from build123d import *
from OCP.BRepFilletAPI import BRepFilletAPI_MakeChamfer

# Parameters (mm, degrees)
BOSS_EXTRUDE1_DEPTH            = 7.5
CUT_EXTRUDE1_REACH             = 58.013
SKETCH2_R                      = 1
CUT_EXTRUDE1_DIRECTION_2_DEPTH = 57.013391256
CHAMFER1_SIZE                  = 5
CHAMFER1_SIZE2                 = 4.351474633
CUT_EXTRUDE2_REACH             = 57.607
SKETCH3_R                      = 13.75
SKETCH11_W                     = 45
SKETCH11_H                     = 7.5
BOSS_EXTRUDE2_DEPTH            = 5
M4_TAPPED_HOLE1_D              = 3.3
CUT_EXTRUDE3_REACH             = 57.607
SKETCH6_R                      = 4.1
M4_TAPPED_HOLE2_REACH          = 61.725
M4_TAPPED_HOLE2_BORE_R         = 1.65
M3_TAPPED_HOLE1_AT_2_COUNT     = 2
M3_TAPPED_HOLE1_AT_2_PITCH     = 12


with BuildPart() as part:
    # Sketch1 → Boss-Extrude1 (new body)
    with BuildSketch(Plane(origin=(0, 0, 0), x_dir=(1, 0, 0), z_dir=(0, 1, 0))):
        Polygon((-22.5, 0), (22.5, 0), (22.5, 14.6), (27.5, 14.6), (32.5, 45), (-32.5, 45), (-27.5, 14.6), (-22.5, 14.6), align=None)
    extrude(amount=BOSS_EXTRUDE1_DEPTH)

    # Sketch2 → Cut-Extrude1 (cut, up to next)
    with BuildSketch(Plane(origin=(0, 7.5, 0), x_dir=(1, 0, 0), z_dir=(0, 1, 0)), mode=Mode.PRIVATE) as cut_extrude1_sk1:
        with Locations((-23.5, 14.6)):
            Circle(SKETCH2_R)
    cut_extrude1_tool1 = extrude(cut_extrude1_sk1.sketch, amount=-CUT_EXTRUDE1_REACH, mode=Mode.PRIVATE) & part.part
    # Sketch2 → Cut-Extrude1 (cut, up to next)
    with BuildSketch(Plane(origin=(0, 7.5, 0), x_dir=(1, 0, 0), z_dir=(0, 1, 0)), mode=Mode.PRIVATE) as cut_extrude1_sk2:
        with Locations((23.5, 14.6)):
            Circle(SKETCH2_R)
    cut_extrude1_tool2 = extrude(cut_extrude1_sk2.sketch, amount=-CUT_EXTRUDE1_REACH, mode=Mode.PRIVATE) & part.part
    add(cut_extrude1_tool1.solids().sort_by_distance((-23.5, 7.5, -14.6))[0], mode=Mode.SUBTRACT)
    add(cut_extrude1_tool2.solids().sort_by_distance((23.5, 7.5, -14.6))[0], mode=Mode.SUBTRACT)

    # Sketch2 → Cut-Extrude1 direction 2 (cut)
    with BuildSketch(Plane(origin=(0, 7.5, 0), x_dir=(1, 0, 0), z_dir=(0, 1, 0))):
        with Locations((-23.5, 14.6)):
            Circle(SKETCH2_R)
        with Locations((23.5, 14.6)):
            Circle(SKETCH2_R)
    extrude(amount=CUT_EXTRUDE1_DIRECTION_2_DEPTH, mode=Mode.SUBTRACT)

    # Chamfer1: one chamfer whose edges measure the first distance from different faces: ONE call of the kernel's chamfer builder (chamfer() names one face for all edges)
    chamfer1_edges_1 = [part.edges().sort_by_distance(p)[0] for p in [
        (-32.5, 3.75, -45),
    ]]
    chamfer1_side_1 = [part.faces().sort_by_distance(p)[0] for p in [
        (0, 3.75, -45),
    ]]
    chamfer1_edges_2 = [part.edges().sort_by_distance(p)[0] for p in [
        (32.5, 3.75, -45),
    ]]
    chamfer1_side_2 = [part.faces().sort_by_distance(p)[0] for p in [
        (30, 3.75, -29.8),
    ]]
    chamfer1 = BRepFilletAPI_MakeChamfer(part.part.solid().wrapped)
    for e in chamfer1_edges_1:
        chamfer1.Add(CHAMFER1_SIZE, CHAMFER1_SIZE2, e.wrapped, chamfer1_side_1[0].wrapped)  # the first distance lies on this face
    for e in chamfer1_edges_2:
        chamfer1.Add(CHAMFER1_SIZE, CHAMFER1_SIZE2, e.wrapped, chamfer1_side_2[0].wrapped)  # the first distance lies on this face
    add(Compound.cast(chamfer1.Shape()), mode=Mode.REPLACE)

    # Sketch3 → Cut-Extrude2 (cut, up to next)
    with BuildSketch(Plane(origin=(0, 7.5, 0), x_dir=(1, 0, 0), z_dir=(0, 1, 0)), mode=Mode.PRIVATE) as cut_extrude2_sk1:
        with Locations(Location((0, 21, 0), (0, 0, 270))):
            Circle(SKETCH3_R)
    cut_extrude2_tool1 = extrude(cut_extrude2_sk1.sketch, amount=-CUT_EXTRUDE2_REACH, mode=Mode.PRIVATE) & part.part
    add(cut_extrude2_tool1.solids().sort_by_distance((0, 7.5, -21))[0], mode=Mode.SUBTRACT)

    # Sketch11 → Boss-Extrude2 (add)
    with BuildSketch(Plane.XY):
        with Locations((0, 3.75)):
            Rectangle(SKETCH11_W, SKETCH11_H)
    extrude(amount=BOSS_EXTRUDE2_DEPTH)

    # M4 Tapped Hole1 (through all)
    with Locations(Plane(origin=(0, 0, 0), x_dir=(-1, 0, 0), z_dir=(0, -1, 0))):
        with Locations((-18.3, 21), (18.3, 21)):
            Hole(M4_TAPPED_HOLE1_D / 2)

    # Sketch6 → Cut-Extrude3 (cut, up to next)
    with BuildSketch(Plane.XZ, mode=Mode.PRIVATE) as cut_extrude3_sk1:
        with Locations(Location((18.5, -28.5, 0), (0, 0, 270))):
            Circle(SKETCH6_R)
    cut_extrude3_tool1 = extrude(cut_extrude3_sk1.sketch, amount=-CUT_EXTRUDE3_REACH, mode=Mode.PRIVATE) & part.part
    # Sketch6 → Cut-Extrude3 (cut, up to next)
    with BuildSketch(Plane.XZ, mode=Mode.PRIVATE) as cut_extrude3_sk2:
        with Locations(Location((-18.5, -28.5, 0), (0, 0, 270))):
            Circle(SKETCH6_R)
    cut_extrude3_tool2 = extrude(cut_extrude3_sk2.sketch, amount=-CUT_EXTRUDE3_REACH, mode=Mode.PRIVATE) & part.part
    add(cut_extrude3_tool1.solids().sort_by_distance((18.5, 0, -28.5))[0], mode=Mode.SUBTRACT)
    add(cut_extrude3_tool2.solids().sort_by_distance((-18.5, 0, -28.5))[0], mode=Mode.SUBTRACT)

    # M4 Tapped Hole2 bore → M4 Tapped Hole2 (cut, up to next)
    with BuildSketch(Plane(origin=(0, 0, -45), x_dir=(-1, 0, 0), z_dir=(0, 0, -1)), mode=Mode.PRIVATE) as m4_tapped_hole2_sk1:
        with Locations((-18.5, 3.75)):
            Circle(M4_TAPPED_HOLE2_BORE_R)
    m4_tapped_hole2_tool1 = extrude(m4_tapped_hole2_sk1.sketch, amount=-M4_TAPPED_HOLE2_REACH, mode=Mode.PRIVATE) & part.part
    # M4 Tapped Hole2 bore → M4 Tapped Hole2 (cut, up to next)
    with BuildSketch(Plane(origin=(0, 0, -45), x_dir=(-1, 0, 0), z_dir=(0, 0, -1)), mode=Mode.PRIVATE) as m4_tapped_hole2_sk2:
        with Locations((18.5, 3.75)):
            Circle(M4_TAPPED_HOLE2_BORE_R)
    m4_tapped_hole2_tool2 = extrude(m4_tapped_hole2_sk2.sketch, amount=-M4_TAPPED_HOLE2_REACH, mode=Mode.PRIVATE) & part.part
    add(m4_tapped_hole2_tool1.solids().sort_by_distance((18.5, 3.75, -45))[0], mode=Mode.SUBTRACT)
    add(m4_tapped_hole2_tool2.solids().sort_by_distance((-18.5, 3.75, -45))[0], mode=Mode.SUBTRACT)

    # Sketch10 → M3 Tapped Hole1 (revolve, cut)
    with BuildSketch(Plane(origin=(22.5, 3.75, -10.5), x_dir=(0, 0, -1), z_dir=(0, 1, 0))):
        Polygon((0, 0), (0, 10.751075774), (1.25, 10), (1.25, 0), align=None)
    m3_tapped_hole1 = revolve(axis=Axis((28.85, 3.75, -10.5), (-1, 0, 0)), mode=Mode.SUBTRACT)

    # M3 Tapped Hole1 at 2: M3 Tapped Hole1 ×2
    with Locations(*[(0, 0, i * M3_TAPPED_HOLE1_AT_2_PITCH) for i in range(1, M3_TAPPED_HOLE1_AT_2_COUNT)]):
        add(m3_tapped_hole1, mode=Mode.SUBTRACT)

    # Mirror1: M3 Tapped Hole1 across plane
    add(m3_tapped_hole1.mirror(Plane(origin=(0, 0, 0), x_dir=(0, 0, 1), z_dir=(1, 0, 0))), mode=Mode.SUBTRACT)

    # Mirror1 copy 1 sketch → Mirror1 copy 1 (revolve, cut)
    with BuildSketch(Plane(origin=(-22.5, 3.75, 1.5), x_dir=(0, 0, -1), z_dir=(0, 1, 0))):
        Polygon((0, 0), (0, -10.751075774), (1.25, -10), (1.25, 0), align=None)
    revolve(axis=Axis((-28.85, 3.75, 1.5), (-1, 0, 0)), mode=Mode.SUBTRACT)


solid = part.part
Can you work these out from the model? Positions are in its coordinate system, mm. A direction names the side the tool comes from. Round coordinates to 2 decimals unless told otherwise and drop trailing zeros. Write each loop counter-clockwise with the first axis right and the second up, starting at its lowest first coordinate (ties: lowest second). Pieces come first, ordered by that corner, then holes. Notation, with made-up numbers: (3, 46.25) - (47, 46.25) arc R17 ccw to (47, 57.25) - close; hole circle Ø9 at (-28, 65.5). An arc over 180 degrees is marked (long way). Write each question's results on one line, items separated by ' | '. Start each with the question number.
1) Please list where these lines run through material, in increasing order: line 1 (X direction, y = 1.5, z = -20); line 2 (X direction, y = 4.25, z = -21); line 3 (Z direction, x = -18.3, y = 2.75).
2) Suppose I cut it at D-D (z = -8.5). List the corners of the cut face in (x, y) for me.
3) We'd pull the mould along X, two halves only. Please class faces 4 (the flat face through (-29.677, 3.698, -27.836)), 5 (the cylindrical face through (23.5, 3.8, -15.6)), 6 (the flat face through (-15, 0, -20)): released by +X, released by -X, zero draft, split by the parting line, or undercut.
4) Suppose I cut it at A-A (x = 0). List the corners of the cut face in (y, z) for me.
5) Suppose I cut it at B-B (z = -30). List the corners of the cut face in (x, y) for me, and give its area (3 significant figures).
6) Which directions (+Z, -Z, +X, -X, +Y, -Y) give clear straight access to the entire face, cutting with the end or side of a thin tool? Please do faces 1 (the flat face through (-22.5, 4, -5)), 2 (the cylindrical face through (19.81, 2.75, -38.72)), 3 (the cylindrical face through (-17.57, 3.7, -9.25)).
7) Suppose I cut it at C-C (x = 18.5). List the corners of the cut face in (y, z) for me.
8) For pin 1 Ø2 at (y, z) = (3.75, -10.5) entering from -X; pin 2 Ø3.5 at (x, y) = (26, 4.5) entering from +Z; pin 3 Ø1.5 at (y, z) = (3.75, 1.5) entering from -X; pin 4 Ø3 at (x, z) = (-18.3, -21) entering from +Y, each with a flat end and sliding along its axis, tell me the tip position at first contact or that it passes through.
Here are the results:
1) line 1: x = -28.39 to -19.61, -16.99 to -13.71, 13.71 to 16.99, 19.61 to 28.39 | line 2: x = -28.55 to -19.95, -16.65 to -13.75, 13.75 to 16.65, 19.95 to 28.55 | line 3: z = -24.4 to -22.65, -19.35 to -11.25, -9.75 to 0.75, 2.25 to 5
2) outline: (-22.5, 0) - (-5.73, 0) - (-5.73, 7.5) - (-22.5, 7.5) - close; (5.73, 0) - (22.5, 0) - (22.5, 7.5) - (5.73, 7.5) - close
3) face 4: released by -X | face 5: undercut | face 6: zero draft
4) outline: (0, -45) - (7.5, -45) - (7.5, -34.75) - (0, -34.75) - close; (0, -7.25) - (7.5, -7.25) - (7.5, 5) - (0, 5) - close
5) outline: (-30.03, 0) - (-22.32, 0) - (-22.32, 7.5) - (-30.03, 7.5) - close; (-14.68, 0) - (-10.4, 0) - (-10.4, 7.5) - (-14.68, 7.5) - close; (10.4, 0) - (14.68, 0) - (14.68, 7.5) - (10.4, 7.5) - close; (22.32, 0) - (30.03, 0) - (30.03, 7.5) - (22.32, 7.5) - close | area: 180 mm2
6) face 1: +Z, -X, +Y, -Y | face 2: -Z | face 3: -X
7) outline: (0, -45) - (2.1, -45) - (2.1, -32.6) - (0, -32.6) - close; (0, -24.4) - (7.5, -24.4) - (7.5, -22.64) - (0, -22.64) - close; (0, -19.36) - (7.5, -19.36) - (7.5, 5) - (0, 5) - close; (5.4, -45) - (7.5, -45) - (7.5, -32.6) - (5.4, -32.6) - close; hole circle Ø2.5 at (3.75, -10.5); hole circle Ø2.5 at (3.75, 1.5)
8) pin 1: stops at x = -12.35 | pin 2: stops at z = -14.6 | pin 3: stops at x = -12.2 | pin 4: passes through
